The listing builds one solid part. Answer for the finished solid, in the listing's coordinates (mm). A direction names the side the tool comes from. Round coordinates to 2 decimals unless told otherwise and drop trailing zeros. Order: outer loops, then holes, each group sorted by start corner. A loop starts at its lowest first (then second) coordinate and runs counter-clockwise, first axis right, second up. Notation, with made-up numbers: (74, -30) -> (119, -30) arc R30 cw to (119, -7) -> close; hole circle Ø8 at (2, 66.5). An arc over 180 degrees is marked (long way). Return JSON: item names as keys, results as strings. Group by question number.
(1) Each of these flat-tipped pins is pushed along its axis until it touches: pin 1 (1.1 mm diameter, centred on x = 0.5, z = 2, fed in from -Y); pin 2 (0.5 mm diameter, centred on x = 2, y = 0, fed in from +Z); pin 3 (1.5 mm diameter, centred on x = -4, z = -9, fed in from +Y). Where does it stop, or does it pass through?
(2) The part is cut by section C-C (x = -7.75). Determine the outline of the cut face in (y, z), plus the area to 3 significant figures.
(3) Which of the six approach directions +Z, -Z, +X, -X, +Y, -Y give full straight-line access (tool end or side, diameter ignored) to faces 1 (the face through (0, 0.5, 2)), 2 (the face through (-0.13, 5.88, -4.81)), 3 (the face through (0, -1.75, 1))?
(4) The part is cut by section A-A (y = 0). Determine the outline of the cut face in (x, z).
(5) Consider line 1 (Z direction, x = -3.25, y = 0); line 2 (Y direction, x = 3.25, z = -3); line 3 (Z direction, x = -8, y = 4.25). Determine where each line is inside the solid, lowest interval first. Write a range as [from, to].
(6) The part is cut by section B-B (z = -8.25). Determine the outline of the cut face in (x, y), plus the area to 3 significant figures.
(7) Determine the mould class of faces 4 (the face through (0.13, -0.27, -1.37)), 5 (the face through (0, -1, 2.5)), 6 (the face through (0, 1.75, 1)) for opening direction Y: +Y half, -Y half, draft (parallel to the pull), parting line (faces both ways), or undercut.
from build123d import *

# Parameters (mm, degrees)
F0_W     = 18
F0_H     = 3.5
F1_DEPTH = 2.5
F3_DEPTH = 1
F4_W     = 18
F4_H     = 3.5
F5_DEPTH = 0.5
F7_DEPTH = 18
F8_R     = 1.25
F9_DEPTH = 18.001


with BuildPart() as f1:
    # F0 (on Top) → F1 (new body)
    with BuildSketch(Plane.XY):
        Rectangle(F0_W, F0_H)
    extrude(amount=F1_DEPTH)

    # F2 (on face) → F3 (cut)
    with BuildSketch(Plane.XY.offset(2.5)):
        with BuildLine():
            ThreePointArc((-8.5, 0), (-8.6464466094, 0.3535533906), (-9, 0.5))
            Line((-9, 0.5), (-9, -0.5))
            ThreePointArc((-9, -0.5), (-8.6464466094, -0.3535533906), (-8.5, 0))
        make_face()
        with BuildLine():
            Line((9, 0.5), (-9, 0.5))
            ThreePointArc((-9, 0.5), (-8.6464466094, 0.3535533906), (-8.5, 0))
            ThreePointArc((-8.5, 0), (-8.6464466094, -0.3535533906), (-9, -0.5))
            Line((-9, -0.5), (9, -0.5))
            ThreePointArc((9, -0.5), (8.5, 0), (9, 0.5))
        make_face()
        with BuildLine():
            Line((-9, -0.5), (-9, 0.5))
            ThreePointArc((-9, 0.5), (-9.5, 0), (-9, -0.5))
        make_face()
        with BuildLine():
            ThreePointArc((9.5, 0), (9.3535533906, 0.3535533906), (9, 0.5))
            Line((9, 0.5), (9, -0.5))
            ThreePointArc((9, -0.5), (9.3535533906, -0.3535533906), (9.5, 0))
        make_face()
        with BuildLine():
            Line((9, -0.5), (9, 0.5))
            ThreePointArc((9, 0.5), (8.5, 0), (9, -0.5))
        make_face()
    extrude(amount=-F3_DEPTH, mode=Mode.SUBTRACT)

    # F4 (on face) → F5 (join)
    with BuildSketch(Plane(origin=(0, 0, 0), x_dir=(1, 0, 0), z_dir=(0, 0, -1))):
        Rectangle(F4_W, F4_H)
    extrude(amount=F5_DEPTH)

    # F6 (on face) → F7 (join)
    with BuildSketch(Plane(origin=(-9, 0, 0), x_dir=(0, -1, 0), z_dir=(-1, 0, 0))):
        with BuildLine():
            ThreePointArc((3.7058600132, -10.71875), (5.3960707964, -8.6234366698), (6, -6))
            ThreePointArc((6, -6), (4.8218253805, -2.4292857857), (1.75, -0.2608798584))
            Line((1.75, -0.2608798584), (1.75, -0.5))
            Line((1.75, -0.5), (-1.75, -0.5))
            Line((-1.75, -0.5), (-1.75, -0.2608798584))
            ThreePointArc((-1.75, -0.2608798584), (-5.897742288, -4.8969878041), (-3.7058600132, -10.71875))
            ThreePointArc((-3.7058600132, -10.71875), (-2.0132976594, -2.1513782851), (5.25, -7))
            ThreePointArc((5.25, -7), (4.8486217149, -9.0132976594), (3.7058600132, -10.71875))
        make_face()
        with BuildLine():
            Line((1.75, -0.5), (1.75, -0.2608798584))
            ThreePointArc((1.75, -0.2608798584), (0, 0), (-1.75, -0.2608798584))
            Line((-1.75, -0.2608798584), (-1.75, -0.5))
            Line((-1.75, -0.5), (1.75, -0.5))
        make_face()
    extrude(amount=-F7_DEPTH)

    # F8 (on face) → F9 (cut, through all)
    with BuildSketch(Plane.YZ.offset(9)):
        with Locations((0, -0.15)):
            Circle(F8_R)
    extrude(amount=-F9_DEPTH, mode=Mode.SUBTRACT)


solid = f1.part
Answer below:
{
 "1": {"pin 1": "stops at y = -1.75", "pin 2": "stops at z = 1.5", "pin 3": "stops at y = 5.56"},
 "2": {"outline": "(-3.71, -10.72) arc R5.25 cw (long way) to (3.71, -10.72) arc R6 ccw to (1.75, -0.26) -> (1.75, 2.5) -> (0.5, 2.5) -> (0.5, 1.5) -> (-0.5, 1.5) -> (-0.5, 2.5) -> (-1.75, 2.5) -> (-1.75, -0.26) arc R6 ccw to start; hole circle Ø2.5 at (0, -0.15)", "area": "31.0 mm²"},
 "3": {"face 1": "+Z, +X, -X", "face 2": "+X, -X, +Y", "face 3": "+Z, +X, -X, -Y"},
 "4": {"outline": "(-9, -1.75) -> (9, -1.75) -> (9, -1.4) -> (-9, -1.4) -> close; (-9, 1.1) -> (9, 1.1) -> (9, 1.5) -> (-9, 1.5) -> close"},
 "5": {"line 1": "z = [-1.75, -1.4], [1.1, 1.5]", "line 2": "y = [-5.2, -3.4], [3.4, 5.2]", "line 3": "z = [-10.24, -10.08], [-3.92, -1.76]"},
 "6": {"outline": "(-9, -5.56) -> (9, -5.56) -> (9, -5.1) -> (-9, -5.1) -> close; (-9, 5.1) -> (9, 5.1) -> (9, 5.56) -> (-9, 5.56) -> close", "area": "16.7 mm²"},
 "7": {"face 4": "undercut", "face 5": "draft", "face 6": "+Y half"}
}
